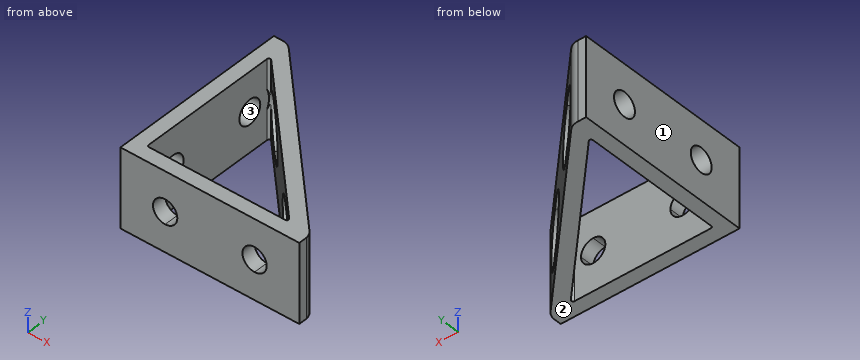
from build123d import *

# Parameters (mm, degrees)
EXTRUDE1_DEPTH     = 22
CUT_EXTRUDE1_DEPTH = 75.054034
CUT_EXTRUDE2_REACH = 76.054
SKETCH5_R          = 6.25
CUT_EXTRUDE3_DEPTH = 75.054186
CUT_EXTRUDE4_REACH = 76.054
SKETCH7_R          = 6.25


with BuildPart() as part:
    # Sketch1 → Extrude1 (new body)
    with BuildSketch(Plane.XY):
        with BuildLine():
            Line((0, 0), (50, 0))
            Line((50, 0), (50, 2.331245))
            ThreePointArc((50, 2.331245), (49.515156, 3.811364), (48.501771, 4.994104))
            Line((48.501771, 4.994104), (5.229403, 48.768941))
            ThreePointArc((5.229403, 48.768941), (3.892255, 49.687806), (2.300146, 50))
            Line((2.300146, 50), (0, 50))
            Line((0, 50), (0, 0))
        make_face()
        with BuildLine():
            Line((4, 43.105797), (4, 4.5))
            ThreePointArc((4, 4.5), (4.146447, 4.146447), (4.5, 4))
            Line((4.5, 4), (42.662662, 4))
            ThreePointArc((42.662662, 4), (43.124047, 4.307326), (43.01825, 4.851507))
            Line((43.01825, 4.851507), (4.855588, 43.457304))
            ThreePointArc((4.855588, 43.457304), (4.309992, 43.568287), (4, 43.105797))
        make_face(mode=Mode.SUBTRACT)
    extrude(amount=EXTRUDE1_DEPTH)

    # Sketch4 → Cut-Extrude1 (cut, through all)
    with BuildSketch(Plane(origin=(0, 50, 0), x_dir=(1, 0, 0), z_dir=(0, 1, 0))):
        with BuildLine():
            ThreePointArc((12.5, -7.6), (9.1, -11), (12.5, -14.4))
            Line((12.5, -14.4), (12.5, -7.6))
        make_face()
        with BuildLine():
            Line((12.5, -7.6), (12.5, -14.4))
            ThreePointArc((12.5, -14.4), (14.904163, -13.404163), (15.9, -11))
            ThreePointArc((15.9, -11), (14.904163, -8.595837), (12.5, -7.6))
        make_face()
        with BuildLine():
            ThreePointArc((37.5, -7.6), (34.1, -11), (37.5, -14.4))
            Line((37.5, -14.4), (37.5, -7.6))
        make_face()
        with BuildLine():
            Line((37.5, -7.6), (37.5, -14.4))
            ThreePointArc((37.5, -14.4), (39.904163, -13.404163), (40.9, -11))
            ThreePointArc((40.9, -11), (39.904163, -8.595837), (37.5, -7.6))
        make_face()
    extrude(amount=-CUT_EXTRUDE1_DEPTH, mode=Mode.SUBTRACT)

    # Cut-Extrude2: up to this face of the body (flat: up to its plane)
    cut_extrude2_end = Plane(part.part.faces().sort_by_distance((23.446976, 4, 11))[0])
    # Sketch5 → Cut-Extrude2 (cut, up to the picked face)
    with BuildSketch(Plane(origin=(0, 50, 0), x_dir=(1, 0, 0), z_dir=(0, 1, 0)), mode=Mode.PRIVATE) as cut_extrude2_sk1:
        with Locations(Location((12.5, -11, 0), (0, 0, 180))):
            Circle(SKETCH5_R)
    cut_extrude2_tool1 = split(extrude(cut_extrude2_sk1.sketch, amount=-CUT_EXTRUDE2_REACH, mode=Mode.PRIVATE), bisect_by=cut_extrude2_end, keep=Keep.BOTH, mode=Mode.PRIVATE)
    # Sketch5 → Cut-Extrude2 (cut, up to the picked face)
    with BuildSketch(Plane(origin=(0, 50, 0), x_dir=(1, 0, 0), z_dir=(0, 1, 0)), mode=Mode.PRIVATE) as cut_extrude2_sk2:
        with Locations(Location((37.5, -11, 0), (0, 0, 325.692636))):
            Circle(SKETCH5_R)
    cut_extrude2_tool2 = split(extrude(cut_extrude2_sk2.sketch, amount=-CUT_EXTRUDE2_REACH, mode=Mode.PRIVATE), bisect_by=cut_extrude2_end, keep=Keep.BOTH, mode=Mode.PRIVATE)
    add(cut_extrude2_tool1.solids().sort_by(Axis((12.5, 50, 11), (0, -1, 0)))[0], mode=Mode.SUBTRACT)
    add(cut_extrude2_tool2.solids().sort_by(Axis((37.5, 50, 11), (0, -1, 0)))[0], mode=Mode.SUBTRACT)

    # Sketch6 → Cut-Extrude3 (cut, through all)
    with BuildSketch(Plane(origin=(50, 0, 0), x_dir=(0, 0, -1), z_dir=(1, 0, 0))):
        with BuildLine():
            ThreePointArc((-7.6, 37.5), (-11, 40.9), (-14.4, 37.5))
            Line((-14.4, 37.5), (-7.6, 37.5))
        make_face()
        with BuildLine():
            Line((-7.6, 37.5), (-14.4, 37.5))
            ThreePointArc((-14.4, 37.5), (-11, 34.1), (-7.6, 37.5))
        make_face()
        with BuildLine():
            ThreePointArc((-7.6, 12.5), (-11, 15.9), (-14.4, 12.5))
            Line((-14.4, 12.5), (-7.6, 12.5))
        make_face()
        with BuildLine():
            Line((-7.6, 12.5), (-14.4, 12.5))
            ThreePointArc((-14.4, 12.5), (-11, 9.1), (-7.6, 12.5))
        make_face()
    extrude(amount=-CUT_EXTRUDE3_DEPTH, mode=Mode.SUBTRACT)

    # Cut-Extrude4: up to this face of the body (flat: up to its plane)
    cut_extrude4_end = Plane(part.part.faces().sort_by_distance((4, 23.69095, 11))[0])
    # Sketch7 → Cut-Extrude4 (cut, up to the picked face)
    with BuildSketch(Plane(origin=(50, 0, 0), x_dir=(0, 0, -1), z_dir=(1, 0, 0)), mode=Mode.PRIVATE) as cut_extrude4_sk1:
        with Locations((-11, 12.5)):
            Circle(SKETCH7_R)
    cut_extrude4_tool1 = split(extrude(cut_extrude4_sk1.sketch, amount=-CUT_EXTRUDE4_REACH, mode=Mode.PRIVATE), bisect_by=cut_extrude4_end, keep=Keep.BOTH, mode=Mode.PRIVATE)
    # Sketch7 → Cut-Extrude4 (cut, up to the picked face)
    with BuildSketch(Plane(origin=(50, 0, 0), x_dir=(0, 0, -1), z_dir=(1, 0, 0)), mode=Mode.PRIVATE) as cut_extrude4_sk2:
        with Locations((-11, 37.5)):
            Circle(SKETCH7_R)
    cut_extrude4_tool2 = split(extrude(cut_extrude4_sk2.sketch, amount=-CUT_EXTRUDE4_REACH, mode=Mode.PRIVATE), bisect_by=cut_extrude4_end, keep=Keep.BOTH, mode=Mode.PRIVATE)
    add(cut_extrude4_tool1.solids().sort_by(Axis((50, 12.5, 11), (-1, 0, 0)))[0], mode=Mode.SUBTRACT)
    add(cut_extrude4_tool2.solids().sort_by(Axis((50, 37.5, 11), (-1, 0, 0)))[0], mode=Mode.SUBTRACT)


solid = part.part
The model under review builds one solid part; all positions refer to its coordinate system, in mm. Face numbers are marked on the shaded views. Round coordinates to 2 decimals unless told otherwise and drop trailing zeros. Loops run counter-clockwise (first coordinate to the right, second up) from the corner with the lowest first, then second, coordinate; pieces in that order, holes last. Notation, with made-up numbers: (27, 21) -> (77, 21) arc R5 cw to (77, 28) -> close; hole circle Ø4 at (77.25, 68). An arc over 180 degrees is marked (long way). One line per question, with ' | ' between items. Start each with the question number.
Item 1: For pin 1 (11 mm diameter, centred on y = 37.5, z = 11, fed in from +X); pin 2 (11 mm diameter, centred on x = 12.5, z = 11, fed in from +Y); pin 3 (2 mm diameter, centred on x = 31, z = 12.5, fed in from +Y), all flat-tipped, find the tip position at first contact; note any pin that passes through.
Item 2: Wall thickness on line 1 along Z through (x, y) = (41, 12.5); line 2 along Z through (x, y) = (1, 37.5); line 3 along X through (y, z) = (28.5, 21.25): over which ranges is each line inside the solid? List them lowest first. Write a range as [from, to].
Item 3: Draft analysis for pull direction Z (two halves, no side actions). For the marked faces 1, 2 and 3, state which applies: +Z half, -Z half, draft (parallel to the pull), parting line (faces both ways), or undercut.
Item 4: Add section B-B, the plane x = 25. Write out the cut boundary in (y, z).
Item 5: Add section A-A, the plane y = 41.5. Write out the cut boundary in (x, z), then the cut area to 3 significant figures.
Return value:
1) pin 1: stops at x = 4 | pin 2: stops at y = 4 | pin 3: stops at y = 23.71
2) line 1: z = [0, 4.75], [17.25, 22] | line 2: z = [0, 7.6], [14.4, 22] | line 3: x = [0, 4], [19.64, 25.27]
3) face 1: draft | face 2: -Z half | face 3: undercut
4) outline: (0, 0) -> (4, 0) -> (4, 22) -> (0, 22) -> close; (23.08, 0) -> (28.77, 0) -> (28.77, 22) -> (23.08, 22) -> close
5) outline: (0, 0) -> (4, 0) -> (4, 22) -> (0, 22) -> close; (6.79, 0) -> (12.41, 0) -> (12.41, 4.75) arc R6.25 cw to (8.5, 6.2) -> (6.79, 6.2) -> close; (6.79, 15.8) -> (8.5, 15.8) arc R6.25 cw to (12.41, 17.25) -> (12.41, 22) -> (6.79, 22) -> close | area: 150 mm2
